Autodesk Inventor part; units mm, degrees
ref_plane "YZ Plane" through (0, 0, 0) normal (1, 0, 0) x (0, 1, 0)
ref_plane "XZ Plane" through (0, 0, 0) normal (0, 1, 0) x (-1, 0, 0)
ref_plane "XY Plane" through (0, 0, 0) normal (0, 0, 1) x (1, 0, 0)
sketch "Sketch1" plane through (0, 0, 0) normal (0, 1, 0) x (-1, 0, 0)
  line L0 (0, 0) -> (-16, 0)
  line L1 (-16, 0) -> (-16, -34)
  line L2 (-16, -34) -> (0, -34)
  line L3 (0, -34) -> (0, 0)
  dimension "d0" = 16
  dimension "d1" = 34
extrude "Extrusion1" add sketch "Sketch1" along normal blind 3
sketch "Sketch2" plane through (0, 3, 0) normal (0, 1, 0) x (1, 0, 0)
  line L0 (0, 0) -> (16, 0)
  line L1 (8, 0) -> (8, 2.5)
  line L2 (16, 34) -> (0, 34)
  line L3 (8, 34) -> (8, 31.5)
  dimension "d4" = 2.5
  dimension "d5" = 2.5
hole "Hole1" at (8, 3, -31.5) at (8, 3, -2.5) direction (0, -1, 0) diameter 4 depth 10 tip angle 118
fillet "Fillet1" radius 0.8 8 edges at (0, 1.5, 0) (0, 1.5, -34) (16, 1.5, 0) (16, 1.5, -34) (16, 3, -17) (8, 3, -34) (0, 3, -17) (8, 3, 0)
Work out the finished part from the listing and answer in its coordinate system (mm). A direction names the side the tool comes from. Give positions to 0.01 mm unless a question says otherwise; leave off trailing zeros. Loops run counter-clockwise (first coordinate to the right, second up) from the corner with the lowest first, then second, coordinate; pieces in that order, holes last. Notation, with made-up numbers: M 77,6.25 L 111,6.25 A8 cw 111,18.25 Z; hole C 13.5,83.25 d3. An arc over 180 degrees is marked long. One line per item, written item: value. Start each with the question number.
1. Determine the mould class of faces 6 (the face through (8, 1, 0)), 7 (the face through (6.017, 1.479, -2.76)), 8 (the face through (0.24, 2.77, -16.77)) for opening direction X: released by +X, released by -X, zero draft, split by the parting line, or undercut.
2. Find section C-C (x = 8.75). State how many separate pieces and enclosed holes the cut face has, and give its area (3 significant figures).
3. Find section B-B (y = 0.45). Give the vertices of the cut face in (x, z), and give its area (3 significant figures).
4. Find section A-A (z = -31.5). Give the vertices of the cut face in (x, y), and give its area (3 significant figures).
5. Find the intervals of material crossed by probe 1 along Z at (x, y) = (8, 1.1); probe 2 along X at (y, z) = (1, -2.5); probe 3 along Z at (x, y) = (9.75, 1.15), in increasing order.
6. Which of the six approach directions +Z, -Z, +X, -X, +Y, -Y give full straight-line access (tool end or side, diameter ignored) to faces 1 (the face through (8, 3, -17)), 2 (the face through (12.17, 2.77, -0.24)), 3 (the face through (8, 1, -34)), 4 (the face through (3.83, 2.77, -33.76)), 5 (the face through (3.92, 2.77, -0.24))?
Reported:
1. face 6: zero draft
1. face 7: undercut
1. face 8: released by -X
2. separate pieces: 3
2. enclosed holes: 0
2. area: 79.5 mm²
3. outline: M 0,-33.2 A0.8 ccw 0.8,-34 L 15.2,-34 A0.8 ccw 16,-33.2 L 16,-0.8 A0.8 ccw 15.2,0 L 0.8,0 A0.8 ccw 0,-0.8 Z; hole C 8,-31.5 d4; hole C 8,-2.5 d4
3. area: 518 mm²
4. outline: M 0,0 L 6,0 L 6,3 L 0.8,3 A0.8 ccw 0,2.2 Z; M 10,0 L 16,0 L 16,2.2 A0.8 ccw 15.2,3 L 10,3 Z
4. area: 35.7 mm²
5. probe 1: z = -34 to -33.5, -29.5 to -4.5, -0.5 to 0
5. probe 2: x = 0 to 6, 10 to 16
5. probe 3: z = -34 to -32.47, -30.53 to -3.47, -1.53 to 0
6. face 1: +Z, -Z, +X, -X, +Y
6. face 2: +Z, +X, +Y
6. face 3: -Z, +X, -X, +Y, -Y
6. face 4: -Z, -X, +Y
6. face 5: +Z, -X, +Y
